```python
from build123d import *

# Parameters (mm, degrees)
F0_W     = 50.8
F0_H     = 63.5
F1_DEPTH = 31.75
F3_DEPTH = 31.75
F4_R     = 6.35
F5_DEPTH = 19.05
F6_R     = 3.175
F7_DEPTH = 25.4


with BuildPart() as f1:
    # F0 (on Front) → F1 (new body)
    with BuildSketch(Plane.XZ):
        with Locations((25.4, 31.75)):
            Rectangle(F0_W, F0_H)
    extrude(amount=F1_DEPTH)

    # F2 (on face) → F3 (cut)
    with BuildSketch(Plane.XZ.offset(31.75)):
        with BuildLine():
            Line((0, 63.5), (0, 6.35))
            ThreePointArc((0, 6.35), (8.980256, 10.069744), (12.7, 19.05))
            Line((12.7, 19.05), (12.7, 50.8))
            ThreePointArc((12.7, 50.8), (16.419744, 59.780256), (25.4, 63.5))
            Line((25.4, 63.5), (0, 63.5))
        make_face()
        with BuildLine():
            ThreePointArc((38.1, 19.05), (41.819744, 10.069744), (50.8, 6.35))
            Line((50.8, 6.35), (50.8, 63.5))
            Line((50.8, 63.5), (25.4, 63.5))
            ThreePointArc((25.4, 63.5), (34.380256, 59.780256), (38.1, 50.8))
            Line((38.1, 50.8), (38.1, 19.05))
        make_face()
    extrude(amount=-F3_DEPTH, mode=Mode.SUBTRACT)

    # F4 (on face) → F5 (cut)
    with BuildSketch(Plane.XZ.offset(31.75)):
        with BuildLine():
            Line((38.1, 19.05), (38.1, 50.8))
            ThreePointArc((38.1, 50.8), (25.4, 38.1), (12.7, 50.8))
            Line((12.7, 50.8), (12.7, 19.05))
            ThreePointArc((12.7, 19.05), (8.980256, 10.069744), (0, 6.35))
            Line((0, 6.35), (50.8, 6.35))
            ThreePointArc((50.8, 6.35), (41.819744, 10.069744), (38.1, 19.05))
        make_face()
        with Locations((25.4, 50.8)):
            Circle(F4_R)
    extrude(amount=-F5_DEPTH, mode=Mode.SUBTRACT)

    # F6 (on face) → F7 (cut)
    with BuildSketch(Plane.XY.offset(6.35)):
        with Locations((6.35, -25.4)):
            Circle(F6_R)
        with BuildLine():
            ThreePointArc((6.35, -31.75), (1.859872, -29.890128), (0, -25.4))
            Line((0, -25.4), (0, -31.75))
            Line((0, -31.75), (6.35, -31.75))
        make_face()
        with Locations((44.45, -25.4)):
            Circle(F6_R)
        with BuildLine():
            ThreePointArc((50.8, -25.4), (48.940128, -29.890128), (44.45, -31.75))
            Line((44.45, -31.75), (50.8, -31.75))
            Line((50.8, -31.75), (50.8, -25.4))
        make_face()
    extrude(amount=-F7_DEPTH, mode=Mode.SUBTRACT)


solid = f1.part
```
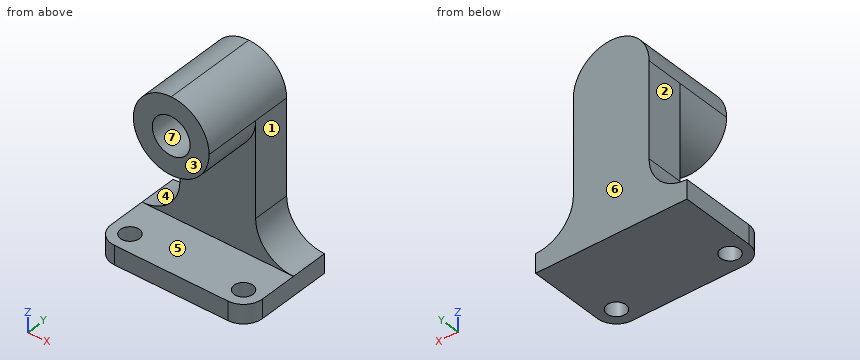
Design review of the part built by this model. Coordinates are the model's own, in mm. Face numbers are marked on the shaded views. A direction names the side the tool comes from. Coordinates: 2 decimals unless noted, no trailing zeros. Loops run counter-clockwise (first coordinate to the right, second up) from the corner with the lowest first, then second, coordinate; pieces in that order, holes last. Notation, with made-up numbers: (47, 84.5) - (95, 84.5) arc R24 ccw to (95, 106.5) - close; hole circle Ø1 at (-24.5, 50.25). An arc over 180 degrees is marked (long way). Use CSV: the item, a comma, the result in double quotes. Start each with the question number.
1) Consider section A-A on y = -17. Write out the cut boundary in (x, z).
2) Wall thickness on L1, parallel to Z at x = 25, y = -26; L2, parallel to Z at x = 28, y = -18; L3, parallel to X at y = -25, z = 5: over which ranges is each line inside the solid? List them lowest first. Write a range as from..to.
3) Consider section D-D on y = -5. Write out the cut boundary in (x, z), then the cut area to 3 significant figures.
4) The part is to be moulded in two halves that separate along Z. For the marked faces 4, 5, 6 and 7, say which applies: +Z half, -Z half, draft (parallel to the pull), parting line (faces both ways), or undercut.
5) For pin 1 Ø6.5 at (x, z) = (26, 48) entering from -Y; pin 2 Ø6 at (x, y) = (39.5, -23) entering from +Z; pin 3 Ø10 at (y, z) = (-6, 42) entering from -X, all flat-tipped, find the tip position at first contact; note any pin that passes through.
6) Consider section B-B on x = 46.5. Write out the cut boundary in (y, z), then the cut area to 3 significant figures.
7) Consider section C-C on z = 49. Write out the cut boundary in (x, y).
8) Tool access review of the marked faces 1, 2 and 3: name each direction out of +Z, -Z, +X, -X, +Y, -Y from which nothing blocks a thin tool from reaching the whole face with its end or side.
Geometry says:
1,outline,"(0, 0) - (50.8, 0) - (50.8, 6.35) - (0, 6.35) - close; circle Ø25.4 at (25.4, 50.8); hole circle Ø12.7 at (25.4, 50.8)"
2,L1,"0..6.35, 38.11..44.46, 57.14..63.49"
2,L2,"0..6.35, 38.37..45.01, 56.59..63.23"
2,L3,"0..3.2, 9.5..41.3, 47.6..50.8"
3,outline,"(0, 0) - (50.8, 0) - (50.8, 6.35) arc R12.7 cw to (38.1, 19.05) - (38.1, 50.8) arc R12.7 ccw to (12.7, 50.8) - (12.7, 19.05) arc R12.7 cw to (0, 6.35) - close"
3,area,"1,770 mm^2"
4,face 4,"+Z half"
4,face 5,"undercut"
4,face 6,"draft"
4,face 7,"undercut"
5,pin 1,"y = -12.7"
5,pin 2,"z = 56.97"
5,pin 3,"x = 12.7"
6,outline,"(-31.41, 0) - (-27.82, 0) - (-27.82, 6.35) - (-31.41, 6.35) - close; (-22.98, 0) - (0, 0) - (0, 7.1) - (-12.7, 7.1) - (-12.7, 6.35) - (-22.98, 6.35) - close"
6,area,"178 mm^2"
7,outline,"(12.7, -12.7) - (12.83, -12.7) - (12.83, -31.75) - (19.31, -31.75) - (19.31, -12.7) - (31.49, -12.7) - (31.49, -31.75) - (37.97, -31.75) - (37.97, -12.7) - (38.1, -12.7) - (38.1, 0) - (12.7, 0) - close"
8,face 1,"+Z, +X, +Y, -Y"
8,face 2,"+Z, -X, +Y, -Y"
8,face 3,"+Z, -Z, +X, -X, -Y"
